Can you work these out from the model? Positions are in its coordinate system, mm. Face numbers are marked on the shaded views. A direction names the side the tool comes from. Coordinates: 2 decimals unless noted, no trailing zeros. Write each loop counter-clockwise with the first axis right and the second up, starting at its lowest first coordinate (ties: lowest second). Pieces come first, ordered by that corner, then holes.
```python
from build123d import *

# Parameters (mm, degrees)
BOSS_EXTRUDE1_DEPTH = 4.7625
BOSS_EXTRUDE2_DEPTH = 5.159375
BOSS_EXTRUDE3_DEPTH = 5.159375
SKETCH4_R           = 1.6637
CUT_EXTRUDE1_DEPTH  = 19.466419322
SKETCH5_W           = 2.38125
SKETCH5_H           = 5.55625
CUT_EXTRUDE2_DEPTH  = 2.38125
EXTRUDE_THIN1_DEPTH = 3.175
CUT_EXTRUDE3_REACH  = 25.891
SKETCH7_W           = 6.35
SKETCH7_H           = 0.79375
SKETCH8_W           = 10.31875
SKETCH8_H           = 0.508
EXTRUDE_THIN2_DEPTH = 3.175
SKETCH9_W           = 5.813488842
SKETCH9_H           = 0.79375
CUT_EXTRUDE4_DEPTH  = 72.39
CUT_EXTRUDE5_REACH  = 32.782
CUT_EXTRUDE6_DEPTH  = 27.884611297
CHAMFER1_SIZE       = 0.762
CHAMFER2_SIZE       = 0.127
SKETCH12_W          = 3.429
SKETCH12_H          = 6.35
CUT_EXTRUDE7_DEPTH  = 1.524
SKETCH13_W          = 2.921
SKETCH13_H          = 5.842
BOSS_EXTRUDE4_DEPTH = 3.96875
FILLET1_RADIUS      = 1.4605
FILLET1_LENGTH      = 5.842
EXTRUDE_THIN5_START = -2.38125
EXTRUDE_THIN5_DEPTH = 4.7625


# Read off the part's stored shape, not the designer's step: Extrude-Thin5
with BuildPart() as part:
    # Sketch1 → Boss-Extrude1 (new, symmetric)
    with BuildSketch(Plane(origin=(0, 0, 0), x_dir=(1, 0, 0), z_dir=(0, 1, 0))):
        with BuildLine():
            Line((-10.715625, 7.9375), (10.715625, 7.9375))
            ThreePointArc((10.715625, 7.9375), (12.399423023, 7.240048023), (13.096875, 5.55625))
            Line((13.096875, 5.55625), (13.096875, -5.55625))
            ThreePointArc((13.096875, -5.55625), (12.399423023, -7.240048023), (10.715625, -7.9375))
            Line((10.715625, -7.9375), (-10.715625, -7.9375))
            ThreePointArc((-10.715625, -7.9375), (-12.399423023, -7.240048023), (-13.096875, -5.55625))
            Line((-13.096875, -5.55625), (-13.096875, 5.55625))
            ThreePointArc((-13.096875, 5.55625), (-12.399423023, 7.240048023), (-10.715625, 7.9375))
        make_face()
    extrude(amount=BOSS_EXTRUDE1_DEPTH, both=True)

    # Sketch2 → Boss-Extrude2 (add, symmetric)
    with BuildSketch(Plane(origin=(0, 0, 0), x_dir=(1, 0, 0), z_dir=(0, 1, 0))):
        with BuildLine():
            Line((7.388225, 7.9375), (10.715625, 7.9375))
            ThreePointArc((10.715625, 7.9375), (12.399423023, 7.240048023), (13.096875, 5.55625))
            Line((13.096875, 5.55625), (13.096875, 2.22885))
            Line((13.096875, 2.22885), (9.769475, 2.22885))
            ThreePointArc((9.769475, 2.22885), (8.085676977, 2.926301977), (7.388225, 4.6101))
            Line((7.388225, 4.6101), (7.388225, 7.9375))
        make_face()
    extrude(amount=BOSS_EXTRUDE2_DEPTH, both=True)

    # Sketch3 → Boss-Extrude3 (add, symmetric)
    with BuildSketch(Plane(origin=(0, 0, 0), x_dir=(1, 0, 0), z_dir=(0, 1, 0))):
        with BuildLine():
            Line((-7.388225, -7.9375), (-10.715625, -7.9375))
            ThreePointArc((-10.715625, -7.9375), (-12.399423023, -7.240048023), (-13.096875, -5.55625))
            Line((-13.096875, -5.55625), (-13.096875, -2.22885))
            Line((-13.096875, -2.22885), (-9.769475, -2.22885))
            ThreePointArc((-9.769475, -2.22885), (-8.085676977, -2.926301977), (-7.388225, -4.6101))
            Line((-7.388225, -4.6101), (-7.388225, -7.9375))
        make_face()
    extrude(amount=BOSS_EXTRUDE3_DEPTH, both=True)

    # Sketch4 → Cut-Extrude1 (cut, through all)
    with BuildSketch(Plane(origin=(0, 5.159375, 0), x_dir=(1, 0, 0), z_dir=(0, 1, 0))):
        with Locations(Location((-10.24255, -5.083175, 0), (0, 0, 270))):
            Circle(SKETCH4_R)
        with Locations(Location((10.24255, 5.083175, 0), (0, 0, 270))):
            Circle(SKETCH4_R)
    extrude(amount=-CUT_EXTRUDE1_DEPTH, mode=Mode.SUBTRACT)

    # Sketch5 → Cut-Extrude2 (cut)
    with BuildSketch(Plane.ZY.offset(13.096875)):
        with Locations((-6.746875, 0)):
            Rectangle(SKETCH5_W, SKETCH5_H)
    extrude(amount=-CUT_EXTRUDE2_DEPTH, mode=Mode.SUBTRACT)

    # Sketch6 → Extrude-Thin1 (add, symmetric)
    with BuildSketch(Plane(origin=(0, 0, 0), x_dir=(1, 0, 0), z_dir=(0, 1, 0))):
        with BuildLine():
            Line((-0.936625, 7.9375), (-0.936625, 10.2235))
            ThreePointArc((-0.936625, 10.2235), (-1.271401949, 11.031723051), (-2.079625, 11.3665))
            Line((-2.079625, 11.3665), (-10.715625, 11.3665))
            Line((-10.715625, 11.3665), (-10.715625, 10.8585))
            Line((-10.715625, 10.8585), (-2.079625, 10.8585))
            ThreePointArc((-2.079625, 10.8585), (-1.630612194, 10.672512806), (-1.444625, 10.2235))
            Line((-1.444625, 10.2235), (-1.444625, 7.9375))
            Line((-1.444625, 7.9375), (-0.936625, 7.9375))
        make_face()
    extrude(amount=EXTRUDE_THIN1_DEPTH, both=True)

    # Sketch7 → Cut-Extrude3 (cut, up to next)
    with BuildSketch(Plane(origin=(0, 0, -11.3665), x_dir=(-1, 0, 0), z_dir=(0, 0, -1)), mode=Mode.PRIVATE) as cut_extrude3_sk1:
        with Locations((7.540625, 2.778125)):
            Rectangle(SKETCH7_W, SKETCH7_H)
    cut_extrude3_tool1 = extrude(cut_extrude3_sk1.sketch, amount=-CUT_EXTRUDE3_REACH, mode=Mode.PRIVATE) & part.part
    cut_extrude3 = cut_extrude3_tool1.solids().sort_by_distance((-7.540625, 2.778125, -11.3665))[0]
    add(cut_extrude3, mode=Mode.SUBTRACT)

    # Sketch8 → Extrude-Thin2 (add, symmetric)
    with BuildSketch(Plane(origin=(0, 0, 0), x_dir=(1, 0, 0), z_dir=(0, 1, 0))):
        with Locations((-18.25625, 3.96875)):
            Rectangle(SKETCH8_W, SKETCH8_H)
        with Locations((-18.25625, -1.5875)):
            Rectangle(SKETCH8_W, SKETCH8_H)
    extrude(amount=EXTRUDE_THIN2_DEPTH, both=True)

    # Sketch9 → Cut-Extrude4 (cut)
    with BuildSketch(Plane(origin=(0, 0, -4.22275), x_dir=(-1, 0, 0), z_dir=(0, 0, -1))):
        with Locations((20.508880579, 2.778125)):
            Rectangle(SKETCH9_W, SKETCH9_H)
    cut_extrude4 = extrude(amount=-CUT_EXTRUDE4_DEPTH, mode=Mode.SUBTRACT)

    # Mirror1: Cut-Extrude3, Cut-Extrude4 across plane
    add(cut_extrude3.mirror(Plane.ZX), mode=Mode.SUBTRACT)
    add(cut_extrude4.mirror(Plane.ZX), mode=Mode.SUBTRACT)

    # Sketch10 → Cut-Extrude5 (cut, up to next)
    with BuildSketch(Plane(origin=(0, 0, -11.3665), x_dir=(-1, 0, 0), z_dir=(0, 0, -1)), mode=Mode.PRIVATE) as cut_extrude5_sk1:
        with BuildLine():
            Line((7.032625, 0.71842049), (7.709958333, 0.478946993))
            ThreePointArc((7.709958333, 0.478946993), (8.048625, 0), (7.709958333, -0.478946993))
            Line((7.709958333, -0.478946993), (7.032625, -0.71842049))
            ThreePointArc((7.032625, -0.71842049), (6.016625, 0), (7.032625, 0.71842049))
        make_face()
    cut_extrude5_tool1 = extrude(cut_extrude5_sk1.sketch, amount=-CUT_EXTRUDE5_REACH, mode=Mode.PRIVATE) & part.part
    add(cut_extrude5_tool1.solids().sort_by_distance((-6.978953, 0, -11.3665))[0], mode=Mode.SUBTRACT)

    # Sketch11 → Cut-Extrude6 (cut, through all)
    with BuildSketch(Plane(origin=(0, 0, -4.22275), x_dir=(-1, 0, 0), z_dir=(0, 0, -1))):
        with BuildLine():
            Line((20.621625, 0.71842049), (21.298958333, 0.478946993))
            ThreePointArc((21.298958333, 0.478946993), (21.637625, 0), (21.298958333, -0.478946993))
            Line((21.298958333, -0.478946993), (20.621625, -0.71842049))
            ThreePointArc((20.621625, -0.71842049), (19.605625, 0), (20.621625, 0.71842049))
        make_face()
    extrude(amount=-CUT_EXTRUDE6_DEPTH, mode=Mode.SUBTRACT)

    # Chamfer1
    chamfer1_edges = [part.edges().sort_by_distance(p)[0] for p in [
        (-10.715625, 2.38125, -11.1125),
        (-23.415625, 2.38125, 1.5875),
        (-23.415625, 2.38125, -3.96875),
        (-10.715625, -2.38125, -11.1125),
        (-23.415625, -2.38125, 1.5875),
        (-23.415625, -2.38125, -3.96875),
    ]]
    chamfer(chamfer1_edges, length=CHAMFER1_SIZE)

    # Chamfer2
    chamfer2_edges = [part.edges().sort_by_distance(p)[0] for p in [
        (-10.715625, 0, -11.3665),
        (-10.715625, 0, -10.8585),
        (-10.334625, -2.00025, -11.3665),
        (-10.334625, 2.00025, -11.3665),
        (-10.334625, -2.00025, -10.8585),
        (-10.334625, 2.00025, -10.8585),
        (-23.415625, 0, 1.3335),
        (-23.034625, 2.00025, 1.3335),
        (-23.034625, -2.00025, 1.3335),
        (-23.415625, 0, 1.8415),
        (-23.034625, 2.00025, 1.8415),
        (-23.034625, -2.00025, 1.8415),
        (-23.415625, 0, -4.22275),
        (-23.415625, 0, -3.71475),
        (-23.034625, -2.00025, -4.22275),
        (-23.034625, 2.00025, -4.22275),
        (-23.034625, -2.00025, -3.71475),
        (-23.034625, 2.00025, -3.71475),
    ]]
    chamfer(chamfer2_edges, length=CHAMFER2_SIZE)

    # Sketch12 → Cut-Extrude7 (cut)
    with BuildSketch(Plane.XY.offset(7.9375)):
        with Locations((7.2517, 0)):
            Rectangle(SKETCH12_W, SKETCH12_H)
    extrude(amount=-CUT_EXTRUDE7_DEPTH, mode=Mode.SUBTRACT)

    # Sketch13 → Boss-Extrude4 (add)
    with BuildSketch(Plane.XY.offset(6.4135)):
        with Locations((7.2517, 0)):
            Rectangle(SKETCH13_W, SKETCH13_H)
    extrude(amount=BOSS_EXTRUDE4_DEPTH)

    # Fillet1: full round fillet: the end face becomes a half cylinder, R = half its width
    fillet1_face = Plane((7.2517, 0, 10.38225), x_dir=(0, -1, 0), z_dir=(0, 0, 1))  # on the end face: x along it, z out of the body
    fillet1_slab = fillet1_face.offset(-FILLET1_RADIUS / 2) * Box(FILLET1_LENGTH, 2 * FILLET1_RADIUS, FILLET1_RADIUS, mode=Mode.PRIVATE)  # the body's end, R deep
    fillet1_round = Plane((7.2517, 0, 8.92175), x_dir=(0, 0, 1), z_dir=(0, -1, 0)) * Cylinder(FILLET1_RADIUS, FILLET1_LENGTH, mode=Mode.PRIVATE)  # its axis R under the face
    add(fillet1_slab - fillet1_round, mode=Mode.SUBTRACT)

    # Sketch14 → Revolve1 (revolve)
    with BuildSketch(Plane(origin=(0, 0, 0), x_dir=(0, 0, -1), z_dir=(1, 0, 0))):
        with BuildLine():
            Line((-5.1562, -4.7625), (-5.1562, -5.581854839))
            ThreePointArc((-5.1562, -5.581854839), (-5.946357191, -5.361015463), (-6.507514618, -4.7625))
            Line((-6.507514618, -4.7625), (-5.1562, -4.7625))
        make_face()
    revolve1 = revolve(axis=Axis((0, -4.7625, 5.1562), (0, -1, 0)))

    # Mirror2: Revolve1 across plane
    add(revolve1.mirror(Plane.ZX))

    # Extrude-Thin5 outline → Extrude-Thin5 (add)
    with BuildSketch(Plane(origin=(0, 0, 0), x_dir=(1, 0, 0), z_dir=(0, 1, 0)).offset(EXTRUDE_THIN5_START)):
        with BuildLine():
            Line((50.755963212, -18.321063831), (50.844036788, -17.82075688))
            Line((50.844036788, -17.82075688), (7.853115161, -10.252674511))
            ThreePointArc((7.853115161, -10.252674511), (6.998488468, -10.360132484), (6.231935352, -9.967283506))
            Line((6.231935352, -9.967283506), (0.463963212, -8.951894987))
            ThreePointArc((0.463963212, -8.951894987), (0.313447508, -8.865036728), (0.254, -8.701741511))
            Line((0.254, -8.701741511), (0.254, -7.9375))
            Line((0.254, -7.9375), (-0.254, -7.9375))
            Line((-0.254, -7.9375), (-0.254, -8.701741511))
            ThreePointArc((-0.254, -8.701741511), (-0.075657476, -9.191627163), (0.375889636, -9.452201938))
            Line((0.375889636, -9.452201938), (50.755963212, -18.321063831))
        make_face()
    extrude(amount=EXTRUDE_THIN5_DEPTH)


solid = part.part
```
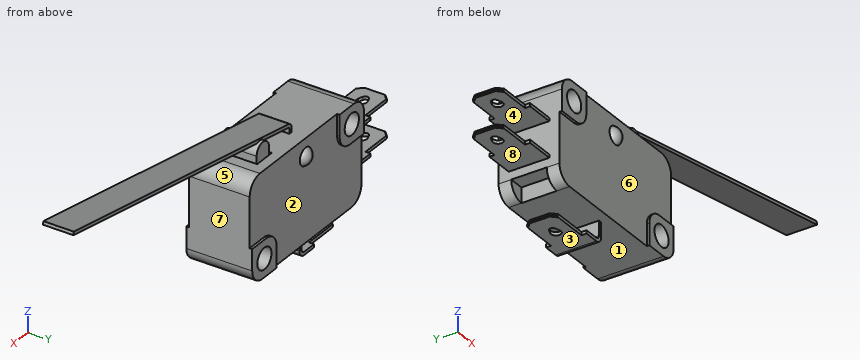
1. We'd pull the mould along Z, two halves only. Please class the marked faces 1, 2 and 3: released by +Z, released by -Z, zero draft, split by the parting line, or undercut.
2. If we section it at A-A, the plane x = 22: List the corners of the cut face in (y, z) for me, plus the area to 3 significant figures.
3. Which directions (+Z, -Z, +X, -X, +Y, -Y) give clear straight access to the entire face, cutting with the end or side of a thin tool? Please do the marked faces 4, 5, 6, 7 and 8.
4. If I drill on L1, parallel to Z at x = -14.5, y = 0; L2, parallel to Z at x = -4.5, y = 0.75; L3, parallel to Z at x = -10, y = -0.25, over which ranges is the centre line in solid material (lowest first)?
5. I'm going to push flat-ended pins straight in: P1, Ø1.7, axis at x = 11, z = -4.5, coming from the +Y side; P2, Ø2, axis at x = 39.5, y = -1, coming from the +Z side; P3, Ø2, axis at x = 25, y = -2.5, coming from the -Z side; P4, Ø1, axis at x = -2.5, z = -10, coming from the -Y side. Where does each tip first touch, or does it pass through?
Answers:
1. face 1: undercut
1. face 2: zero draft
1. face 3: released by -Z
2. outline: (-2.38, 12.74) - (2.38, 12.74) - (2.38, 13.26) - (-2.38, 13.26) - close
2. area: 2.46 mm2
3. face 4: -X, +Y, -Y
3. face 5: +X, +Y, -Y
3. face 6: -Y
3. face 7: -Z, +X, +Y, -Y
3. face 8: -Z, -X, +Y, -Y
4. L1: z = -4.22 to -3.71, 1.33 to 1.84
4. L2: z = -11.37 to -10.86, -7.94 to 7.94
4. L3: z = -11.37 to -10.86, -7.94 to 3.44, 6.73 to 7.94
5. P1: stops at y = 5.16
5. P2: stops at z = 16.52
5. P3: stops at z = 13.1
5. P4: passes through
